Autodesk Fusion 360 part; units mm, degrees
sketch "Sketch1" plane through (0, 0, 0) normal (0, 0, 1) x (1, 0, 0)
  circle A0 centre (-15.1, 66.4157) radius 3.6
  circle A1 centre (15.1, 66.4157) radius 3.6
  line L0 (-21.35, -67.8157) -> (-21.35, -65.0157)
  arc A2 (-21.35, -65.0157) -> (-28.55, -65.0157) centre (-24.95, -65.0157) ccw
  line L1 (-28.55, -65.0157) -> (-28.55, -67.8157)
  arc A3 (-28.55, -67.8157) -> (-21.35, -67.8157) centre (-24.95, -67.8157) ccw
  line L2 (-24.95, -67.8157) -> (-24.95, -65.0157) construction
  line L3 (28.55, -67.8157) -> (28.55, -65.0157)
  arc A4 (28.55, -65.0157) -> (21.35, -65.0157) centre (24.95, -65.0157) ccw
  line L4 (21.35, -65.0157) -> (21.35, -67.8157)
  arc A5 (21.35, -67.8157) -> (28.55, -67.8157) centre (24.95, -67.8157) ccw
  line L5 (24.95, -67.8157) -> (24.95, -65.0157) construction
  line L6 (21.35, -66.4157) -> (-21.35, -66.4157) construction
  line L7 (0, 0) -> (0, -66.4157) construction
  line L8 (0, 0) -> (0, 66.4157) construction
  line L9 (-11.5, 66.4157) -> (11.5, 66.4157) construction
  line L10 (11.5, 62.5719) -> (11.5, 70.0303) construction
  line L11 (-11.5, 69.0679) -> (-11.5, 63.414) construction
  line L12 (-21.5, 77.0157) -> (21.5, 77.0157)
  line L13 (21.5, 77.0157) -> (34, -79.4157)
  line L14 (34, -79.4157) -> (-34, -79.4157)
  line L15 (-34, -79.4157) -> (-21.5, 77.0157)
  line L16 (-30.5341, -76.2157) -> (-18.5455, 73.8157)
  line L17 (-18.5455, 73.8157) -> (18.5455, 73.8157)
  line L18 (18.5455, 73.8157) -> (30.5341, -76.2157)
  line L19 (30.5341, -76.2157) -> (-30.5341, -76.2157)
  line L20 (-23.194, 55.8157) -> (23.194, 55.8157)
  line L21 (-32.0023, -54.4157) -> (32.0023, -54.4157)
  line L22 (-23.4497, 52.6157) -> (23.4497, 52.6157)
  line L23 (-31.7466, -51.2157) -> (31.7466, -51.2157)
  point P0 (-24.95, -66.4157)
  point P1 (24.95, -66.4157)
  dimension "d1" = 7.2
  dimension "d2" = 7.2
  dimension "d3" = 7.2
  dimension "d4" = 7.2
  dimension "d5" = 10
  dimension "d6" = 10
  dimension "d8" = 42.7
  dimension "d9" = 23
  dimension "d10" = 124.6
  dimension "d11" = 43
  dimension "d12" = 21.5
  dimension "d13" = 68
  dimension "d14" = 34
  dimension "d15" = 7
  dimension "d16" = 8
  dimension "d17" = 3.2
  dimension "d19" = 7
  dimension "d20" = 7
  dimension "d23" = 3.2
  dimension "d24" = 3.2
extrude "Extrude1" add sketch "Sketch1" along normal blind 8 contours A0 | A1 | L0 A2 L1 A3 | L3 A4 L4 A5 | L12 L13 L15 L16 L17 L18 L20 | L15 L16 L20 L22 | L13 L18 L20 L22 | L15 L16 L22 L23 | L16 L17 L18 L20 | L13 L18 L22 L23 | L15 L16 L21 L23 | L13 L18 L21 L23 | L13 L14 L15 L16 L18 L19 L21 | L16 L18 L19 L21
extrude "Extrude5" add sketch "Sketch1" along normal blind 2.4 from surface at 8 contours A0 | A1 | L0 A2 L1 A3 | L3 A4 L4 A5 | L12 L13 L15 L16 L17 L18 L20 | L15 L16 L20 L22 | L13 L18 L20 L22 | L15 L16 L22 L23 | L16 L18 L20 L22 | L16 L17 L18 L20 | L13 L18 L22 L23 | L15 L16 L21 L23 | L16 L18 L22 L23 | L13 L18 L21 L23 | L13 L14 L15 L16 L18 L19 L21 | L16 L18 L21 L23 | L16 L18 L19 L21
fillet "Fillet2" radius 8 4 edges at (-34, -79.4157, 5.2) (34, -79.4157, 5.2) (21.5, 77.0157, 5.2) (-21.5, 77.0157, 5.2)
chamfer "Chamfer3" distance 1 distance2 2 8 edges at (-27.6991, -0.5628, 10.4) (-31.2131, -76.8426, 10.4) (0, -79.4157, 10.4) (31.2131, -76.8426, 10.4) (27.6991, -0.5628, 10.4) (19.5406, 74.8935, 10.4) (0, 77.0157, 10.4) (-19.5406, 74.8935, 10.4) measured on face at (7.3628, -23.968, 10.4) measured on face at (-25.7019, -79.4073, 3.4667) measured on face at (7.3628, -23.968, 10.4) measured on face at (33.246, -72.6073, 3.4667) measured on face at (7.3628, -23.968, 10.4) measured on face at (20.0972, 74.326, 6.9333) measured on face at (7.3628, -23.968, 10.4) measured on face at (-20.8196, 73.3782, 3.4667)
sketch "Sketch3" plane through (0, 0, 0) normal (1, 0, 0) x (0, 1, 0)
  line L0 (66.4157, 0) -> (58.8029, 23.4298)
  line L1 (-66.4157, 0) -> (-75.3617, 27.5331)
  line L2 (-67.8157, 0) -> (-65.0157, 0)
  line L3 (70.0157, 0) -> (62.8157, 0)
  dimension "d47" = 72
  dimension "d50" = 72
ref_plane "WorkPlane1" through (0, 60.3722, 18.6001) normal (0, -0.309, 0.9511) x (1, 0, 0)
sketch "Sketch4" plane through (0, 60.3722, 18.6001) normal (0, -0.309, 0.9511) x (1, 0, 0)
  ellipse E0 centre (15.1, 0) end of major axis (18.7, 0) minor radius 3.4238
  ellipse E1 centre (-15.1, 0) end of major axis (-11.5, 0) minor radius 3.4238
  circle A0 centre (15.1, 0) radius 3.7
  circle A1 centre (-15.1, 0) radius 3.7
  dimension "d64" = 7.4
  dimension "d65" = 7.4
extrude "Extrude6" cut sketch "Sketch4" against normal through all contours E0 | E1 | A0 | A1
ref_plane "WorkPlane2" through (0, -74.6951, 25.4815) normal (0, -0.309, 0.9511) x (1, 0, 0)
sketch "Sketch5" plane through (0, -74.6951, 25.4815) normal (0, -0.309, 0.9511) x (1, 0, 0)
  line L0 (28.65, -1.4) -> (28.65, 1.4)
  arc A0 (28.65, 1.4) -> (21.25, 1.4) centre (24.95, 1.4) ccw
  line L1 (21.25, 1.4) -> (21.25, -1.4)
  arc A1 (21.25, -1.4) -> (28.65, -1.4) centre (24.95, -1.4) ccw
  line L2 (24.95, -1.4) -> (24.95, 1.4) construction
  line L3 (-21.25, -1.4) -> (-21.25, 1.4)
  arc A2 (-21.25, 1.4) -> (-28.65, 1.4) centre (-24.95, 1.4) ccw
  line L4 (-28.65, 1.4) -> (-28.65, -1.4)
  arc A3 (-28.65, -1.4) -> (-21.25, -1.4) centre (-24.95, -1.4) ccw
  line L5 (-24.95, -1.4) -> (-24.95, 1.4) construction
  point P0 (24.95, 0)
  point P1 (-24.95, 0)
  point P2 (24.95, 0)
  point P3 (-24.95, 0)
  dimension "d69" = 7.4
  dimension "d70" = 7.4
  dimension "d71" = 10.2
  dimension "d72" = 10.2
extrude "Extrude7" cut sketch "Sketch5" against normal through all
sketch "Sketch6" plane through (0, 60.3722, 18.6001) normal (0, -0.309, 0.9511) x (1, 0, 0)
  ellipse E0 centre (-15.1, 0) end of major axis (-11.5, 0) minor radius 3.4238
  ellipse E1 centre (15.1, 0) end of major axis (18.7, 0) minor radius 3.4238
  circle A0 centre (-15.1, 0) radius 5.5
  circle A1 centre (15.1, 0) radius 5.5
  dimension "d75" = 11
  dimension "d76" = 11
extrude "Extrude8" cut sketch "Sketch6" against normal blind 10.603 contours E0 | E1 | A0 | A1
sketch "Sketch7" plane through (0, -74.6951, 25.4815) normal (0, -0.309, 0.9511) x (1, 0, 0)
  arc A0 (-21.25, 1.4) -> (-28.65, 1.4) centre (-24.95, 1.4) ccw
  line L0 (-21.25, -1.4) -> (-21.25, 1.4)
  arc A1 (-28.65, -1.4) -> (-21.25, -1.4) centre (-24.95, -1.4) ccw
  line L1 (-28.65, 1.4) -> (-28.65, -1.4)
  arc A2 (28.65, 1.4) -> (21.25, 1.4) centre (24.95, 1.4) ccw
  line L2 (21.25, 1.4) -> (21.25, -1.4)
  arc A3 (21.25, -1.4) -> (28.65, -1.4) centre (24.95, -1.4) ccw
  line L3 (28.65, -1.4) -> (28.65, 1.4)
  line L4 (-19.95, -1.4) -> (-19.95, 1.4)
  arc A4 (-19.95, 1.4) -> (-29.95, 1.4) centre (-24.95, 1.4) ccw
  line L5 (-29.95, 1.4) -> (-29.95, -1.4)
  arc A5 (-29.95, -1.4) -> (-19.95, -1.4) centre (-24.95, -1.4) ccw
  line L6 (29.95, -1.4) -> (29.95, 1.4)
  arc A6 (29.95, 1.4) -> (19.95, 1.4) centre (24.95, 1.4) ccw
  line L7 (19.95, 1.4) -> (19.95, -1.4)
  arc A7 (19.95, -1.4) -> (29.95, -1.4) centre (24.95, -1.4) ccw
  dimension "d79" = 1.3
  dimension "d80" = 10
  dimension "d81" = 1.3
extrude "Extrude9" cut sketch "Sketch7" against normal blind 18.2266 contours A0 L0 A1 L1 | A2 L2 A3 L3 | L4 A4 L5 A5 | L6 A6 L7 A7
equation "d2 = d1"
equation "d12 = d11 / 2"
equation "d14 = d13 / 2"
equation "d17 = ( 0.4 * 8 ) * 1 mm"
equation "d23 = d17"
equation "d24 = d17"
equation "d47 = 90 deg - 18 deg"
equation "d50 = d47"
equation "d64 = d65"
equation "d70 = d69"
equation "d72 = d71"
equation "d76 = d75"
equation "d81 = d79"
Check sheet for the modelled part. Datum: model origin and axes. Units: mm. A direction names the side the tool comes from. Coordinates: 2 decimals unless noted, no trailing zeros. Write each loop counter-clockwise with the first axis right and the second up, starting at its lowest first coordinate (ties: lowest second). Pieces come first, ordered by that corner, then holes.
Item 1: Access from +Z, -Z, +X, -X, +Y, -Y to the whole of each face (thin tool, end or side, straight path). Record for faces 3 (the face through (21.25, -68, 4)), 4 (the face through (-24.45, -0.07, 3.94)), 5 (the face through (19.95, -69, 9)), 6 (the face through (0, 77.016, 4)).
Numbers:
face 3: none
face 4: -Z
face 5: +Z
face 6: +Z, -Z, +X, -X, +Y
Item 2: Mould release check, pull along Y, two halves, no side actions. Record for faces 1 (the face through (19.074, 74.502, 9.608)), 2 (the face through (29.95, -69, 9)): released by +Y, released by -Y, zero draft, split by the parting line, or undercut.
Numbers:
face 1: released by +Y
face 2: undercut
Item 3: Cross-section at C-C on z = 3. Count the separate pieces of the cut face and the enclosed holes in it, then the cut area to 3 significant figures.
Numbers:
separate pieces: 1
enclosed holes: 5
area: 3,030 mm2
Item 4: Scan lines: probe 1 along Y at (x, z) = (4.5, 1); probe 2 along Y at (x, z) = (-17, 3); probe 3 along Z at (x, y) = (-7, -48.5). Record each from-to range of solid material in increasing order.
Numbers:
probe 1: y = -79.42 to -54.42, 55.82 to 77.02
probe 2: y = -79.42 to -54.42, 55.82 to 62.1, 68.78 to 76.48
probe 3: z = 8 to 10.4
Item 5: Cross-section at A-A on x = 8. Record the boundary of the cut face in (y, z).
Numbers:
outline: (-79.42, 0) - (-54.42, 0) - (-54.42, 8) - (55.82, 8) - (55.82, 0) - (77.02, 0) - (77.02, 8.4) - (76.02, 10.4) - (-78.42, 10.4) - (-79.42, 8.4) - close
Item 6: Depth check by flat-ended pin: pin 1 Ø2 at (y, z) = (-69, 9) entering from -X; pin 2 Ø1.3 at (y, z) = (-69, 9) entering from +X; pin 3 Ø6 at (x, y) = (5.5, -2) entering from -Z; pin 4 Ø6 at (x, z) = (-1, 8.5) entering from -Y. Enter the tip coordinate at first touch or a pass-through.
Numbers:
pin 1: stops at x = -33.23
pin 2: stops at x = 33.19
pin 3: stops at z = 8
pin 4: stops at y = -79.42
Item 7: Cross-section at B-B on y = 21. Record the boundary of the cut face in (x, z).
Numbers:
outline: (-25.98, 0) - (-22.77, 0) - (-22.77, 8) - (22.77, 8) - (22.77, 0) - (25.98, 0) - (25.98, 8.4) - (24.97, 10.4) - (-24.97, 10.4) - (-25.98, 8.4) - close
